```python
from build123d import *

# Parameters (mm, degrees)
SKETCH_1_R      = 7.5
SKETCH_1_R_2    = 3.75
EXTRUDE_1_DEPTH = 7
SKETCH_2_R      = 6
EXTRUDE_2_DEPTH = 3
FILLET_1_R      = 2.5


with BuildPart() as part:
    # Эскиз1 → Бобышка-Вытянуть1 (new body)
    with BuildSketch(Plane(origin=(0, 0, 0), x_dir=(1, 0, 0), z_dir=(0, 1, 0))):
        Circle(SKETCH_1_R)
        Circle(SKETCH_1_R_2, mode=Mode.SUBTRACT)
    extrude(amount=-EXTRUDE_1_DEPTH)

    # Эскиз2 → Бобышка-Вытянуть2 (add)
    with BuildSketch(Plane(origin=(0, -7, 0), x_dir=(-1, 0, 0), z_dir=(0, -1, 0))):
        Circle(SKETCH_2_R)
    extrude(amount=-EXTRUDE_2_DEPTH)

    # Скругление1
    fillet_1_edges = [part.edges().sort_by_distance(p)[0] for p in [
        (-7.5, -7, 0),
    ]]
    fillet(fillet_1_edges, radius=FILLET_1_R)


solid = part.part
```
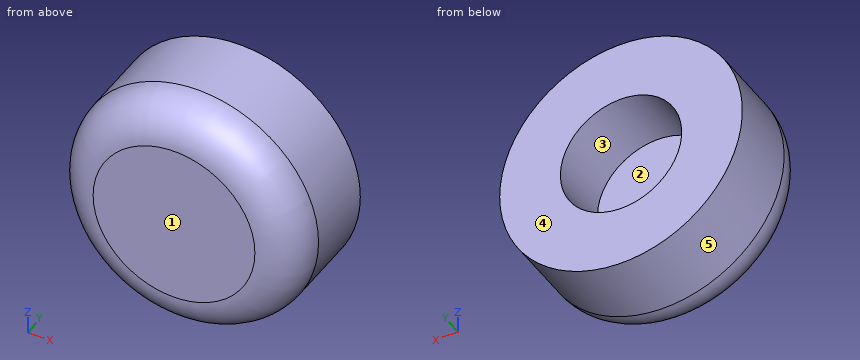
CAD build for the part. Positions are in the model's coordinates, mm. Face numbers are marked on the shaded views. A direction names the side the tool comes from. Give positions to 0.01 mm unless a question says otherwise; leave off trailing zeros. Loops run counter-clockwise (first coordinate to the right, second up) from the corner with the lowest first, then second, coordinate; pieces in that order, holes last. Notation, with made-up numbers: (75.5, 52) -> (85.5, 52) arc R19 ccw to (85.5, 66) -> close; hole circle Ø5 at (13.25, -28). An arc over 180 degrees is marked (long way). Use a Markdown table: item, result.
1. Slice it at C-C (y = -0.5). List the corners of the cut face in (x, z).
Check result:
| item | result |
|---|---|
| outline | circle Ø15 at (0, 0); hole circle Ø7.5 at (0, 0) |
2. Flat gauge pins, fed straight in: pin 1 (2 mm diameter, centred on y = -3, z = 4.5, fed in from -X); pin 2 (2 mm diameter, centred on y = -1.5, z = -6, fed in from +X); pin 3 (4 mm diameter, centred on y = -4, z = -5, fed in from +X). Where does each tip first touch, or does it go through?
Check result:
| item | result |
|---|---|
| pin 1 | stops at x = -6.63 |
| pin 2 | stops at x = 5.59 |
| pin 3 | stops at x = 6.87 |
3. Mould opens along X. For the marked faces 3, 4 and 5 say: pulls with the +X half, pulls with the -X half, needs draft (parallel to the pull), parting line crosses it, or undercut.
Check result:
| item | result |
|---|---|
| face 3 | undercut |
| face 4 | needs draft |
| face 5 | parting line crosses it |
4. Slice it at A-A (x = 0). List the corners of the cut face in (y, z).
Check result:
| item | result |
|---|---|
| outline | (-7, -5) arc R2.5 ccw to (-4.5, -7.5) -> (0, -7.5) -> (0, -3.75) -> (-4, -3.75) -> (-4, 3.75) -> (0, 3.75) -> (0, 7.5) -> (-4.5, 7.5) arc R2.5 ccw to (-7, 5) -> close |
5. Which spindle directions (+Z, -Z, +X, -X, +Y, -Y) get a long thin tool onto all of the face, cutting with end or side? Do the marked faces 1 and 2. Say none if no direction does.
Check result:
| item | result |
|---|---|
| face 1 | +Z, -Z, +X, -X, -Y |
| face 2 | +Y |
6. Slice it at B-B (z = 0). List the corners of the cut face in (x, y), plus the area to 3 significant figures.
Check result:
| item | result |
|---|---|
| outline | (-7.5, -4.5) arc R2.5 ccw to (-5, -7) -> (5, -7) arc R2.5 ccw to (7.5, -4.5) -> (7.5, 0) -> (3.75, 0) -> (3.75, -4) -> (-3.75, -4) -> (-3.75, 0) -> (-7.5, 0) -> close |
| area | 72.3 mm^2 |
7. Wall check: L1, parallel to X at y = -2.2, z = 0; L2, parallel to Y at x = -1, z = 0. Give the ranges that are in metal, low to high. Write a range as [from, to].
Check result:
| item | result |
|---|---|
| L1 | x = [-7.5, -3.75], [3.75, 7.5] |
| L2 | y = [-7, -4] |
8. Slice it at D-D (y = -6). List the corners of the cut face in (x, z), plus the area to 3 significant figures.
Check result:
| item | result |
|---|---|
| outline | circle Ø14 at (0, 0) |
| area | 154 mm^2 |
